Build history of the part. All positions in model axes, mm. A direction names the side the tool comes from. Give positions to 0.01 mm unless a question says otherwise; leave off trailing zeros. Order: outer loops, then holes, each group sorted by start corner. A loop starts at its lowest first (then second) coordinate and runs counter-clockwise, first axis right, second up. Notation, with made-up numbers: M -18,85.5 L 10,85.5 A9 ccw 10,98.5 Z; hole C -20.5,-4.75 d3. An arc over 180 degrees is marked long. Answer as CSV lines item,"result".
from build123d import *

# Parameters (mm, degrees)
SKETCH_W        = 25
SKETCH_H        = 150
PAD_DEPTH       = 6.5
SKETCH001_R     = 1.6
POCKET_DEPTH    = 10
SKETCH002_R     = 1.6
POCKET001_DEPTH = 10
SKETCH003_W     = 5.8
SKETCH003_H     = 3
POCKET002_DEPTH = 6.5
FILLET_R        = 0.4
FILLET001_R     = 0.2
POCKET003_DEPTH = 5
FILLET002_R     = 1
FILLET003_R     = 0.2


with BuildPart() as part:
    # Sketch → Pad (new body)
    with BuildSketch(Plane.XY):
        Rectangle(SKETCH_W, SKETCH_H)
    extrude(amount=PAD_DEPTH)

    # Sketch001 (on Face3 of Pad) → Pocket (cut)
    with BuildSketch(Plane.XZ.offset(75)):
        with Locations((-7.5, 3.25)):
            Circle(SKETCH001_R)
        with Locations((7.5, 3.25)):
            Circle(SKETCH001_R)
    extrude(amount=-POCKET_DEPTH, mode=Mode.SUBTRACT)

    # Sketch002 (on Face1 of Pocket) → Pocket001 (cut)
    with BuildSketch(Plane(origin=(0, 75, 0), x_dir=(-1, 0, 0), z_dir=(0, 1, 0))):
        with Locations((-7.5, 3.25)):
            Circle(SKETCH002_R)
        with Locations((7.5, 3.25)):
            Circle(SKETCH002_R)
    extrude(amount=-POCKET001_DEPTH, mode=Mode.SUBTRACT)

    # Sketch003 (on Face4 of Pocket001) → Pocket002 (cut)
    with BuildSketch(Plane.XY.offset(6.5)):
        with Locations((-7.5, 70.5)):
            Rectangle(SKETCH003_W, SKETCH003_H)
        with Locations((7.5, 70.5)):
            Rectangle(SKETCH003_W, SKETCH003_H)
        with Locations((-7.5, -70.5)):
            Rectangle(SKETCH003_W, SKETCH003_H)
        with Locations((7.5, -70.5)):
            Rectangle(SKETCH003_W, SKETCH003_H)
    extrude(amount=-POCKET002_DEPTH, mode=Mode.SUBTRACT)

    # Fillet
    fillet_edges = [part.edges().sort_by_distance(p)[0] for p in [
        (-12.5, -75, 3.25),
        (12.5, -75, 3.25),
        (12.5, 75, 3.25),
        (-12.5, 75, 3.25),
    ]]
    fillet(fillet_edges, radius=FILLET_R)

    # Fillet001
    fillet001_edges = [part.edges().sort_by_distance(p)[0] for p in [
        (-10.4, 72, 3.25),
        (4.6, 72, 3.25),
        (-10.4, -69, 3.25),
        (4.6, -69, 3.25),
        (-4.6, -69, 3.25),
        (10.4, -69, 3.25),
        (-4.6, 72, 3.25),
        (10.4, 72, 3.25),
        (10.4, 69, 3.25),
        (-4.6, 69, 3.25),
        (10.4, -72, 3.25),
        (-4.6, -72, 3.25),
        (-10.4, -72, 3.25),
        (4.6, -72, 3.25),
        (-10.4, 69, 3.25),
        (4.6, 69, 3.25),
    ]]
    fillet(fillet001_edges, radius=FILLET001_R)

    # Sketch004 (on Face42 of Fillet001) → Pocket003 (cut)
    with BuildSketch(Plane.XY.offset(6.5)):
        Polygon((-10, -60), (-10, 60), (-4.5, 60), (-4.5, 50), (10, 50), (10, -50), (-4.5, -50), (-4.5, -60), align=None)
    extrude(amount=-POCKET003_DEPTH, mode=Mode.SUBTRACT)

    # Fillet002
    fillet002_edges = [part.edges().sort_by_distance(p)[0] for p in [
        (-4.5, 50, 4),
        (10, 50, 4),
        (-4.5, -50, 4),
        (10, -50, 4),
    ]]
    fillet(fillet002_edges, radius=FILLET002_R)

    # Fillet003
    fillet003_edges = [part.edges().sort_by_distance(p)[0] for p in [
        (-4.5, 60, 4),
        (-10, 60, 4),
        (-4.5, -60, 4),
        (-10, -60, 4),
    ]]
    fillet(fillet003_edges, radius=FILLET003_R)


solid = part.part
Item 1: Drop flat-ended pins along their axis: pin 1 (2 mm diameter, centred on x = 1, y = 18, fed in from +Z); pin 2 (1 mm diameter, centred on x = -7, z = 3.5, fed in from -Y); pin 3 (3 mm diameter, centred on x = -7.5, z = 3.25, fed in from +Y). Give the stop position or say it passes through.
Geometry says:
pin 1,"stops at z = 1.5"
pin 2,"stops at y = -65"
pin 3,"stops at y = 65"
Item 2: Pull direction Y, two halves, no side cores. Call faces 5 (the flat face through (7, -65, 3)), 6 (the cylindrical face through (8.77, 67.03, 2.28)), 7 (the flat face through (4.6, -71, 3)): released by +Y, released by -Y, zero draft, split by the parting line, or undercut.
Geometry says:
face 5,"released by -Y"
face 6,"zero draft"
face 7,"undercut"
Item 3: Probe line 1 along Y through (x, z) = (10.25, 0.5); line 2 along X through (y, z) = (-7.5, 3.25); line 3 along Z through (x, y) = (-7.5, 74.2). List the from-to ranges inside material, lowest first. Write a range as from..to.
Geometry says:
line 1,"y = -75..-71.99, -69.01..69.01, 71.99..75"
line 2,"x = -12.5..-10, 10..12.5"
line 3,"z = 0..1.65, 4.85..6.5"
Item 4: Band-saw the part on B-B (y = -46.5). Give the cut face in (x, z).
Geometry says:
outline,"M -12.5,0 L 12.5,0 L 12.5,6.5 L 10,6.5 L 10,1.5 L -10,1.5 L -10,6.5 L -12.5,6.5 Z"
Item 5: Band-saw the part on C-C (x = 0.25). Give the cut face in (y, z), and give its area (3 significant figures).
Geometry says:
outline,"M -75,0 L 75,0 L 75,6.5 L 50,6.5 L 50,1.5 L -50,1.5 L -50,6.5 L -75,6.5 Z"
area,"475 mm2"
Item 6: Band-saw the part on A-A (x = -7.5). State how many separate pieces and enclosed holes the cut face has, and give its area (3 significant figures).
Geometry says:
separate pieces,"5"
enclosed holes,"0"
area,"291 mm2"
Item 7: 3-axis set-ups, long thin cutter, end or side, ignore diameter. For faces 1 (the cylindrical face through (-6.23, 67.03, 2.28)), 2 (the flat face through (-4.5, 55, 4)), 3 (the flat face through (7, 72, 5)), 4 (the cylindrical face through (-8.77, -73.52, 2.28)): which of +Z, -Z, +X, -X, +Y, -Y reach the whole face in a straight line?
Geometry says:
face 1,"+Y"
face 2,"+Z"
face 3,"+Z, -Z"
face 4,"-Y"
